Geometry: final body of the model. Coordinates: model frame, mm. A direction names the side the tool comes from. Coordinates: 2 decimals unless noted, no trailing zeros. Write each loop counter-clockwise with the first axis right and the second up, starting at its lowest first coordinate (ties: lowest second). Pieces come first, ordered by that corner, then holes. Notation, with made-up numbers: (72, -39.5) - (91, -39.5) arc R34 ccw to (91, -6.5) - close; hole circle Ø7 at (30, -15.75). An arc over 180 degrees is marked (long way). Put each result on its own line as item: value.
```python
from build123d import *

# Parameters (mm, degrees)
SKETCH_1_W          = 45
SKETCH_1_H          = 45
SKETCH_1_W_2        = 35
SKETCH_1_H_2        = 35
EXTRUDE_1_DEPTH     = 5
CUT_EXTRUDE_1_DEPTH = 3
SKETCH_3_R          = 0.5
EXTRUDE_2_DEPTH     = 2
SKETCH_4_W          = 5
SKETCH_4_H          = 15
EXTRUDE_3_DEPTH     = 20
SKETCH_5_W          = 5
SKETCH_5_H          = 5
EXTRUDE_4_DEPTH     = 4
SKETCH_6_R          = 1.5
EXTRUDE_5_DEPTH     = 4


with BuildPart() as part:
    # 草圖1 → 填料-伸長1 (new body)
    with BuildSketch(Plane.XY):
        Rectangle(SKETCH_1_W, SKETCH_1_H)
        Rectangle(SKETCH_1_W_2, SKETCH_1_H_2, mode=Mode.SUBTRACT)
    extrude(amount=EXTRUDE_1_DEPTH)

    # 草圖2 → 除料-伸長1 (cut)
    with BuildSketch(Plane.ZY.offset(22.5)):
        with BuildLine():
            Line((2.5, -17.5), (5, -17.5))
            Line((5, -17.5), (5, -22.5))
            Line((5, -22.5), (0, -22.5))
            Line((0, -22.5), (0, -20))
            ThreePointArc((0, -20), (0.732233047, -18.232233047), (2.5, -17.5))
        make_face()
    cut_extrude_1 = extrude(amount=-CUT_EXTRUDE_1_DEPTH, mode=Mode.SUBTRACT)

    # 鏡射1: 除料-伸長1 across plane
    add(cut_extrude_1.mirror(Plane(origin=(0, 0, 0), x_dir=(0, 0, 1), z_dir=(1, 0, 0))), mode=Mode.SUBTRACT)

    # 草圖3 → 填料-伸長2 (add)
    with BuildSketch(Plane.ZY.offset(19.5)):
        with Locations(Location((2.5, -20, 0), (0, 0, 270))):
            Circle(SKETCH_3_R)
    extrude_2 = extrude(amount=EXTRUDE_2_DEPTH)

    # 鏡射2: 填料-伸長2 across plane
    add(extrude_2.mirror(Plane(origin=(0, 0, 0), x_dir=(0, 0, 1), z_dir=(1, 0, 0))))

    # 草圖4 → 填料-伸長3 (add)
    with BuildSketch(Plane.XY.offset(5)):
        with Locations((20, 15)):
            Rectangle(SKETCH_4_W, SKETCH_4_H)
    extrude(amount=EXTRUDE_3_DEPTH)

    # 草圖5 → 填料-伸長4 (add)
    with BuildSketch(Plane.XY.offset(25)):
        with Locations((20, 10)):
            Rectangle(SKETCH_5_W, SKETCH_5_H)
    extrude(amount=EXTRUDE_4_DEPTH)

    # 草圖6 → 填料-伸長5 (add)
    with BuildSketch(Plane.XZ.offset(-7.5)):
        with Locations(Location((20, 27, 0), (0, 0, 90))):
            Circle(SKETCH_6_R)
    extrude(amount=EXTRUDE_5_DEPTH)


solid = part.part
```
1. Section query D-D (z = 27). Return loops of the section in (x, y), then the cut area to 3 significant figures.
Answer below:
outline: (17.5, 7.5) - (18.5, 7.5) - (18.5, 3.5) - (21.5, 3.5) - (21.5, 7.5) - (22.5, 7.5) - (22.5, 12.5) - (17.5, 12.5) - close
area: 37.0 mm²
2. Set-up query: faces 1 (the flat face through (0, -17.5, 2)), 2 (the cylindrical face through (18.99, 5.53, 25.89)), 3 (the flat face through (20, 18, 25)). Return all of +Z, -Z, +X, -X, +Y, -Y with unobstructed straight access to the full face (end or side cutting, diameter ignored); none if empty.
Answer below:
face 1: +Z, -Z
face 2: -Y
face 3: +Z, +X, -X, +Y
3. Section query B-B (y = 6). Return loops of the section in (x, z).
Answer below:
outline: (-22.5, 0) - (-17.5, 0) - (-17.5, 5) - (-22.5, 5) - close; (17.5, 0) - (22.5, 0) - (22.5, 5) - (17.5, 5) - close; circle Ø3 at (20, 27)
4. Mould query, pull axis Y, two halves, no side actions, for faces 4 (the flat face through (0, 17.5, 2)), 5 (the flat face through (20, 12.5, 27)), 6 (the flat face through (-22.5, 1, 2)). Classes: +Y half, -Y half, draft (parallel to the pull), parting line (faces both ways), or undercut.
Answer below:
face 4: undercut
face 5: +Y half
face 6: draft
5. Section query A-A (y = 16). Return loops of the section in (x, z).
Answer below:
outline: (-22.5, 0) - (-17.5, 0) - (-17.5, 5) - (-22.5, 5) - close; (17.5, 0) - (22.5, 0) - (22.5, 25) - (17.5, 25) - close
6. Section query C-C (x = -9.5). Return loops of the section in (y, z).
Answer below:
outline: (-22.5, 0) - (-17.5, 0) - (-17.5, 5) - (-22.5, 5) - close; (17.5, 0) - (22.5, 0) - (22.5, 5) - (17.5, 5) - close
7. Ray query, probe 1 along Y at (x, z) = (-4, 1.75); probe 2 along X at (y, z) = (14.5, 6.5); probe 3 along Z at (x, y) = (-19, 1). Return the intervals inside material, ascending. Write a range as from..to.
Answer below:
probe 1: y = -22.5..-17.5, 17.5..22.5
probe 2: x = 17.5..22.5
probe 3: z = 0..5
8. Pin query (flat end, axial travel): pin 1 Ø4 at (x, z) = (19.5, 12.5) entering from -Y; pin 2 Ø12 at (x, y) = (17, -12) entering from +Z; pin 3 Ø8 at (y, z) = (15.5, 19.5) entering from -X. Return the tip coordinate at first contact, or that it passes through.
Answer below:
pin 1: stops at y = 7.5
pin 2: stops at z = 5
pin 3: stops at x = 17.5
